Autodesk Inventor part; units mm, degrees
ref_plane "YZ Plane" through (0, 0, 0) normal (1, 0, 0) x (0, 1, 0)
ref_plane "XZ Plane" through (0, 0, 0) normal (0, 1, 0) x (-1, 0, 0)
ref_plane "XY Plane" through (0, 0, 0) normal (0, 0, 1) x (1, 0, 0)
sketch "Sketch1" plane through (0, 0, 0) normal (0, 0, 1) x (1, 0, 0)
  line L0 (-22.943, -21.4569) -> (193.057, -21.4569)
  line L1 (-22.943, -21.4569) -> (-12.943, -21.4569)
  line L2 (-12.943, -21.4569) -> (-2.943, -21.4569)
  line L3 (-2.943, -21.4569) -> (-2.943, -64.1369)
  line L4 (-22.943, -21.4569) -> (184.057, -21.4569)
  line L5 (184.057, -21.4569) -> (184.057, -54.3769)
  line L6 (184.057, -54.3769) -> (-2.943, -64.1369)
  line L7 (-12.943, -21.4569) -> (-2.943, -64.1369)
  line L8 (184.057, -21.4569) -> (184.057, 33.1531)
  line L9 (-22.943, -21.4569) -> (-22.943, 89.8331)
  line L10 (-22.943, 89.8331) -> (184.057, 33.1531)
  line L11 (184.057, 33.1531) -> (184.057, 34.1531)
  line L12 (184.057, 34.1531) -> (193.057, 31.6888)
  line L13 (193.057, -21.4569) -> (193.057, 31.6888)
  line L14 (184.057, -54.3769) -> (193.057, -53.9072)
  line L15 (193.057, -21.4569) -> (193.057, -53.9072)
  line L16 (-22.943, -21.4569) -> (-32.943, -21.4569)
  line L17 (-32.943, -21.4569) -> (-42.943, -21.4569)
  line L18 (-22.943, -21.4569) -> (-229.943, -21.4569)
  line L19 (-229.943, -21.4569) -> (-229.943, -54.3769)
  line L20 (-42.943, -21.4569) -> (-42.943, -64.1369)
  line L21 (-229.943, -54.3769) -> (-42.943, -64.1369)
  line L22 (-32.943, -21.4569) -> (-42.943, -64.1369)
  line L23 (-238.943, -21.4569) -> (-238.943, -53.9072)
  line L24 (-229.943, -54.3769) -> (-238.943, -53.9072)
  line L25 (-22.943, -21.4569) -> (-238.943, -21.4569)
  line L26 (-238.943, -21.4569) -> (-238.943, 31.6888)
  line L27 (-229.943, 34.1531) -> (-238.943, 31.6888)
  line L28 (-229.943, -21.4569) -> (-229.943, 33.1531)
  line L29 (-229.943, 33.1531) -> (-229.943, 34.1531)
  line L30 (-22.943, 89.8331) -> (-229.943, 33.1531)
  point P0 (0, 0)
  dimension "d0" = 216
  dimension "d1" = 10
  dimension "d2" = 10
  dimension "d3" = 42.68
  dimension "d4" = 207
  dimension "d5" = 32.92
  dimension "d6" = 54.61
  dimension "d7" = 111.29
  dimension "d8" = 1
extrude "Extrusion1" add sketch "Sketch1" along normal mid plane 5.7 contours L0 L3 L7 | L0 L5 L6 L3
chamfer "Chamfer1" distance 6 angle 25 1 edges at (85.557, -21.4569, -2.85) measured on face at (56.057, -35.6836, -2.85)
fillet "Fillet1" radius 2 1 edges at (90.557, -59.2569, 2.85)
fillet "Fillet2" radius 2 1 edges at (90.557, -59.2569, -2.85)
chamfer "Chamfer2" distance 6 angle 25 1 edges at (85.557, -21.4569, 2.85) measured on face at (55.9024, -35.0241, 2.85)
Geometry check sheet. Reference: the model listing, model coordinates, mm. Round coordinates to 2 decimals unless told otherwise and drop trailing zeros. Order: outer loops, then holes, each group sorted by start corner. A loop starts at its lowest first (then second) coordinate and runs counter-clockwise, first axis right, second up. Notation, with made-up numbers: M 8.25,19.25 L 25.25,19.25 A23 ccw 25.25,52.25 Z; hole C -8.75,23 d11. An arc over 180 degrees is marked long. Answer as CSV lines item,"result".
1) Gauge pin test, flat ends, axial feed: pin 1 Ø5 at (x, y) = (129.5, -56.5) entering from -Z; pin 2 Ø2 at (x, z) = (115, -1.5) entering from -Y. Record the tip position at first contact, or that the pin passes through.
Entries:
pin 1,"z = -2.85"
pin 2,"y = -58.02"
2) Sectioned sample at A-A on y = -40.5. Record the cut outline in (x, z).
Entries:
outline,"M -8.48,-2.85 L 184.06,-2.85 L 184.06,2.85 L -8.48,2.85 Z"
3) Thickness scan on probe 1 along X at (y, z) = (-27.5, -0.45); probe 2 along Z at (x, y) = (40.5, -60); probe 3 along Y at (x, z) = (141, 1.75). Record the ranges inside material, lowest first. Write a range as [from, to].
Entries:
probe 1,"[-11.53, 184.06]"
probe 2,"[-2.85, 2.85]"
probe 3,"[-56.41, -25.1]"
